Geometry: final body of the model. Coordinates: model frame, mm. Face numbers are marked on the shaded views. A direction names the side the tool comes from. Give positions to 0.01 mm unless a question says otherwise; leave off trailing zeros. Write each loop counter-clockwise with the first axis right and the second up, starting at its lowest first coordinate (ties: lowest second). Pieces come first, ordered by that corner, then holes. Notation, with made-up numbers: (72, 52) -> (120, 52) arc R13 cw to (120, 60) -> close; hole circle Ø9 at (73, -8). An arc over 180 degrees is marked (long way). Use CSV: the item, a comma, the result in double quotes. Start each with the question number.
1) Section A-A (z = 0). Output: boundary loops of the cut face in (x, y).
2) Draft query along Z for the marked faces 6, 7, 8 and 9. Return one class per face: pulls with the +Z half, pulls with the -Z half, needs draft (parallel to the pull), parting line crosses it, or undercut.
3) Material intervals for line 1 (X direction, y = -1, z = 0); line 2 (Y direction, x = 12, z = 6.25); line 3 (X direction, y = 3.75, z = -4), sorted ascending. Write a range as [from, to].
4) Contact query for flat-ended pins moving along their axis: P1, Ø1.5, axis at x = 0.5, y = 3.5, coming from the +Z side; P2, Ø8.5, axis at y = 5, z = 1.5, coming from the +X side; P3, Ø1.5, axis at x = -10, y = 8.5, coming from the +Z side. Output: stop coordinate, or through.
5) Section C-C (x = -13.6). Output: boundary loops of the cut face in (y, z), plus the area to 3 significant figures.
6) Section D-D (y = 10.5). Output: boundary loops of the cut face in (x, z), plus the area to 3 significant figures.
7) Set-up query: the marked faces 1, 2, 3, 4 and 5. Return all of +Z, -Z, +X, -X, +Y, -Y with unobstructed straight access to the full face (end or side cutting, diameter ignored); none if empty.
8) Section B-B (y = 2). Output: boundary loops of the cut face in (x, z), plus the area to 3 significant figures.
```python
from build123d import *

# Parameters (mm, degrees)
SKETCH_1_R               = 1.6
EXTRUDE_1_DEPTH          = 2.5
EXTRUDE_2_DEPTH          = 10
EXTRUDE_2_DEPTH_BACK     = 10
CUT_EXTRUDE_START        = 12
SKETCH_4_R               = 25
CUT_EXTRUDE_3_DEPTH      = 12
CUT_EXTRUDE_4_DEPTH      = 12
CUT_EXTRUDE_4_DEPTH_BACK = 12
SKETCH_5_R               = 9


with BuildPart() as part:
    # Sketch 1 → Extrude 1 (new body)
    with BuildSketch(Plane(origin=(0, 0, 0), x_dir=(1, 0, 0), z_dir=(0, 1, 0))):
        with BuildLine():
            Line((16.235294118, -4.941176471), (5.647058824, -10.588235294))
            ThreePointArc((5.647058824, -10.588235294), (0, -12), (-5.647058824, -10.588235294))
            Line((-5.647058824, -10.588235294), (-16.235294118, -4.941176471))
            ThreePointArc((-16.235294118, -4.941176471), (-19.2, 0), (-16.235294118, 4.941176471))
            Line((-16.235294118, 4.941176471), (-5.647058824, 10.588235294))
            ThreePointArc((-5.647058824, 10.588235294), (0, 12), (5.647058824, 10.588235294))
            Line((5.647058824, 10.588235294), (16.235294118, 4.941176471))
            ThreePointArc((16.235294118, 4.941176471), (19.2, 0), (16.235294118, -4.941176471))
        make_face()
        with Locations(Location((-13.6, 0, 0), (0, 0, 270))):
            Circle(SKETCH_1_R, mode=Mode.SUBTRACT)
        with Locations(Location((13.6, 0, 0), (0, 0, 270))):
            Circle(SKETCH_1_R, mode=Mode.SUBTRACT)
    extrude(amount=-EXTRUDE_1_DEPTH)

    # Sketch 2 → Extrude 2 (add, two sides: drawn at the far end of the back side and taken through both)
    with BuildSketch(Plane(origin=(0, 0, 0), x_dir=(0, 0, -1), z_dir=(1, 0, 0)).offset(-EXTRUDE_2_DEPTH_BACK)):
        Polygon((12, 0), (-12, 0), (-7, 5), (-7, 17), (7, 17), (7, 5), align=None)
    extrude(amount=EXTRUDE_2_DEPTH + EXTRUDE_2_DEPTH_BACK)

    # Sketch 4 → Cut-Extrude 3 (cut)
    with BuildSketch(Plane(origin=(0, 0, 0), x_dir=(1, 0, 0), z_dir=(0, 1, 0)).offset(CUT_EXTRUDE_START)):
        Circle(SKETCH_4_R)
        with BuildLine():
            Line((5.647058824, -10.588235294), (10, -8.266666667))
            Line((10, -8.266666667), (16.235294118, -4.941176471))
            ThreePointArc((16.235294118, -4.941176471), (19.2, 0), (16.235294118, 4.941176471))
            Line((16.235294118, 4.941176471), (10, 8.266666667))
            Line((10, 8.266666667), (5.647058824, 10.588235294))
            ThreePointArc((5.647058824, 10.588235294), (2.9104275, 11.641710002), (0, 12))
            ThreePointArc((0, 12), (-2.9104275, 11.641710002), (-5.647058824, 10.588235294))
            Line((-5.647058824, 10.588235294), (-10, 8.266666667))
            Line((-10, 8.266666667), (-16.235294118, 4.941176471))
            ThreePointArc((-16.235294118, 4.941176471), (-19.2, 0), (-16.235294118, -4.941176471))
            Line((-16.235294118, -4.941176471), (-10, -8.266666667))
            Line((-10, -8.266666667), (-5.647058824, -10.588235294))
            ThreePointArc((-5.647058824, -10.588235294), (-2.9104275, -11.641710002), (0, -12))
            ThreePointArc((0, -12), (2.9104275, -11.641710002), (5.647058824, -10.588235294))
        make_face(mode=Mode.SUBTRACT)
    extrude(amount=-CUT_EXTRUDE_3_DEPTH, mode=Mode.SUBTRACT)

    # Sketch 5 → Cut-Extrude 4 (cut, two sides: drawn at the far end of the back side and taken through both)
    with BuildSketch(Plane.XY.offset(-CUT_EXTRUDE_4_DEPTH_BACK)):
        with Locations((0, 17)):
            Circle(SKETCH_5_R)
    extrude(amount=CUT_EXTRUDE_4_DEPTH + CUT_EXTRUDE_4_DEPTH_BACK, mode=Mode.SUBTRACT)


solid = part.part
```
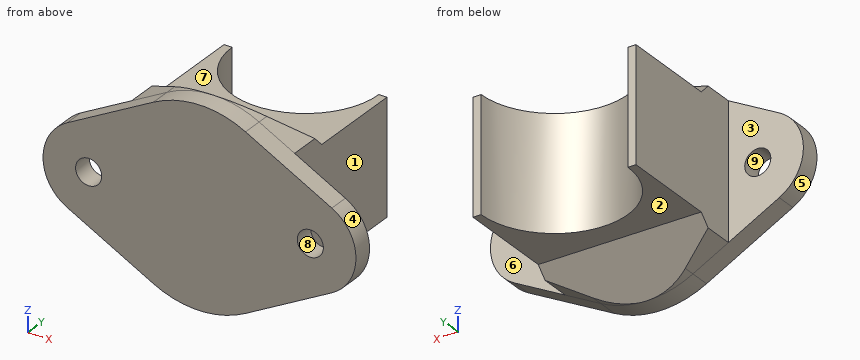
Answers follow:
1,outline,"(-19.2, -2.5) -> (-15.2, -2.5) -> (-15.2, 0) -> (-19.2, 0) -> close; (-12, -2.5) -> (12, -2.5) -> (12, 0) -> (10, 0) -> (10, 17) -> (9, 17) arc R9 cw to (-9, 17) -> (-10, 17) -> (-10, 0) -> (-12, 0) -> close; (15.2, -2.5) -> (19.2, -2.5) -> (19.2, 0) -> (15.2, 0) -> close"
2,face 6,"needs draft"
2,face 7,"pulls with the +Z half"
2,face 8,"undercut"
2,face 9,"undercut"
3,line 1,"x = [-19.2, -15.2], [-12, 12], [15.2, 19.2]"
3,line 2,"y = [-2.5, 0]"
3,line 3,"x = [-10, 10]"
4,P1,"stops at z = 9.25"
4,P2,"stops at x = 10"
4,P3,"stops at z = 7"
5,outline,"(-2.5, -6.35) -> (0, -6.35) -> (0, -1.6) -> (-2.5, -1.6) -> close; (-2.5, 1.6) -> (0, 1.6) -> (0, 6.35) -> (-2.5, 6.35) -> close"
5,area,"23.7 mm^2"
6,outline,"(-10, -7) -> (-6.22, -7) -> (-6.22, 7) -> (-10, 7) -> close; (6.22, -7) -> (10, -7) -> (10, 7) -> (6.22, 7) -> close"
6,area,"106 mm^2"
7,face 1,"+Z, -Z, +X, +Y"
7,face 2,"-Z, +X, -X, +Y"
7,face 3,"+Z, -Z, -X, +Y"
7,face 4,"+X, +Y, -Y"
7,face 5,"-X, +Y, -Y"
8,outline,"(-10, -8.27) -> (-6.75, -10) -> (6.75, -10) -> (10, -8.27) -> (10, 8.27) -> (6.75, 10) -> (-6.75, 10) -> (-10, 8.27) -> close"
8,area,"389 mm^2"
